Read the model definition and answer for the solid it produces. Units are mm, in the model's axes. Round coordinates to 2 decimals unless told otherwise and drop trailing zeros. Write each loop counter-clockwise with the first axis right and the second up, starting at its lowest first coordinate (ties: lowest second). Pieces come first, ordered by that corner, then holes. Notation, with made-up numbers: (45.25, 4) -> (63.25, 4) arc R9 ccw to (63.25, 12) -> close; hole circle Ø8 at (36, 24). An arc over 180 degrees is marked (long way). Return JSON: item names as keys, results as strings. Group by question number.
(1) A cutting plane is placed at D-D on y = 257. Give the vertices of the cut face in (x, z).
(2) A cutting plane is placed at A-A on x = -258.5. Give the vertices of the cut face in (y, z).
(3) Straight lines are drawn through the part: line 1 (X direction, y = 264, z = 1.8); line 2 (X direction, y = 268, z = 0.65); line 3 (X direction, y = 292, z = 2.3). For each, find the intervals that lie inside material, in ascending order.
(4) A cutting plane is placed at B-B on x = -199.5. Give the vertices of the cut face in (y, z), then the cut area to 3 significant figures.
(5) A cutting plane is placed at C-C on z = 1.3. State how many separate pieces and enclosed holes the cut face has, then the cut area to 3 significant figures.
(6) Given pin 1 (3 mm diameter, centred on x = -203.49, y = 292.5, fed in from +Z) (3 decimals); pin 2 (1.5 mm diameter, centred on x = -223.5, z = 1, fed in from +Y); pin 3 (1.5 mm diameter, centred on y = 314, z = 1, fed in from -X); pin 4 (1.5 mm diameter, centred on y = 309.5, z = 1.5, fed in from -X), each flat-ended and moving along its own axis, determine where each tip first touches the part or whether it passes through.
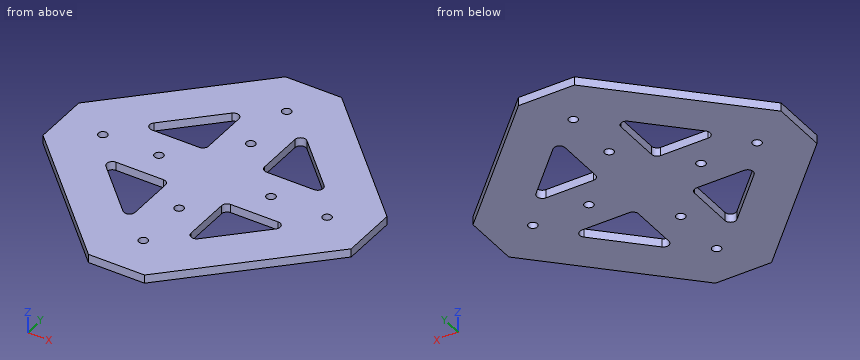
```python
from build123d import *

# Parameters (mm, degrees)
EXTRUDE1_DEPTH     = 3
SKETCH2_R          = 1.6
CUT_EXTRUDE1_DEPTH = 3
EXTRUDE2_DEPTH     = 10


with BuildPart() as part:
    # Sketch1 → Extrude1 (new body)
    with BuildSketch(Plane.XY):
        Polygon((-253.489921235, 347.497048214), (-233.489921235, 347.497048214), (-188.489921235, 302.497048214), (-188.489921235, 282.497048214), (-233.489921235, 237.497048214), (-253.489921235, 237.497048214), (-298.489921235, 282.497048214), (-298.489921235, 302.497048214), align=None)
    extrude(amount=EXTRUDE1_DEPTH)

    # Sketch2 → Cut-Extrude1 (cut)
    with BuildSketch(Plane.XY.offset(3)):
        with Locations((-203.489921235, 292.497048214)):
            Circle(SKETCH2_R)
        with Locations((-223.489921235, 292.497048214)):
            Circle(SKETCH2_R)
        with Locations((-243.489921235, 252.497048214)):
            Circle(SKETCH2_R)
        with Locations((-243.489921235, 272.497048214)):
            Circle(SKETCH2_R)
        with Locations((-283.489921235, 292.497048214)):
            Circle(SKETCH2_R)
        with Locations((-263.489921235, 292.497048214)):
            Circle(SKETCH2_R)
        with Locations((-243.489921235, 312.497048214)):
            Circle(SKETCH2_R)
        with Locations((-243.489921235, 332.497048214)):
            Circle(SKETCH2_R)
    extrude(amount=-CUT_EXTRUDE1_DEPTH, mode=Mode.SUBTRACT)

    # Sketch3 → Extrude2 (cut)
    with BuildSketch(Plane.XY.offset(3)):
        with BuildLine():
            Line((-256.904134797, 322.869631216), (-273.862504237, 305.911261776))
            ThreePointArc((-273.862504237, 305.911261776), (-274.29604974, 303.731681349), (-272.448290675, 302.497048214))
            Line((-272.448290675, 302.497048214), (-255.489921235, 302.497048214))
            ThreePointArc((-255.489921235, 302.497048214), (-254.075707673, 303.082834651), (-253.489921235, 304.497048214))
            Line((-253.489921235, 304.497048214), (-253.489921235, 321.455417653))
            ThreePointArc((-253.489921235, 321.455417653), (-254.72455437, 323.303176718), (-256.904134797, 322.869631216))
        make_face()
        with BuildLine():
            Line((-233.489921235, 304.497048214), (-233.489921235, 321.455417653))
            ThreePointArc((-233.489921235, 321.455417653), (-232.2552881, 323.303176718), (-230.075707673, 322.869631216))
            Line((-230.075707673, 322.869631216), (-213.117338233, 305.911261776))
            ThreePointArc((-213.117338233, 305.911261776), (-212.68379273, 303.731681349), (-214.531551795, 302.497048214))
            Line((-214.531551795, 302.497048214), (-231.489921235, 302.497048214))
            ThreePointArc((-231.489921235, 302.497048214), (-232.904134797, 303.082834651), (-233.489921235, 304.497048214))
        make_face()
        with BuildLine():
            Line((-230.075707673, 262.124465212), (-213.117338233, 279.082834651))
            ThreePointArc((-213.117338233, 279.082834651), (-212.68379273, 281.262415078), (-214.531551795, 282.497048214))
            Line((-214.531551795, 282.497048214), (-231.489921235, 282.497048214))
            ThreePointArc((-231.489921235, 282.497048214), (-232.904134797, 281.911261776), (-233.489921235, 280.497048214))
            Line((-233.489921235, 280.497048214), (-233.489921235, 263.538678774))
            ThreePointArc((-233.489921235, 263.538678774), (-232.2552881, 261.690919709), (-230.075707673, 262.124465212))
        make_face()
        with BuildLine():
            Line((-253.489921235, 280.497048214), (-253.489921235, 263.538678774))
            ThreePointArc((-253.489921235, 263.538678774), (-254.72455437, 261.690919709), (-256.904134797, 262.124465212))
            Line((-256.904134797, 262.124465212), (-273.862504237, 279.082834651))
            ThreePointArc((-273.862504237, 279.082834651), (-274.29604974, 281.262415078), (-272.448290675, 282.497048214))
            Line((-272.448290675, 282.497048214), (-255.489921235, 282.497048214))
            ThreePointArc((-255.489921235, 282.497048214), (-254.075707673, 281.911261776), (-253.489921235, 280.497048214))
        make_face()
    extrude(amount=-EXTRUDE2_DEPTH, mode=Mode.SUBTRACT)


solid = part.part
```
Checks:
{
 "1": {"outline": "(-272.99, 0) -> (-213.99, 0) -> (-213.99, 3) -> (-272.99, 3) -> close"},
 "2": {"outline": "(242.51, 0) -> (263.72, 0) -> (263.72, 3) -> (242.51, 3) -> close; (282.5, 0) -> (302.5, 0) -> (302.5, 3) -> (282.5, 3) -> close; (321.27, 0) -> (342.49, 0) -> (342.49, 3) -> (321.27, 3) -> close"},
 "3": {"line 1": "x = -279.99 to -258.78, -253.49 to -233.49, -228.2 to -206.99", "line 2": "x = -283.99 to -262.78, -253.49 to -233.49, -224.2 to -202.99", "line 3": "x = -298.49 to -285.01, -281.97 to -265.01, -261.97 to -225.01, -221.97 to -205.01, -201.97 to -188.49"},
 "4": {"outline": "(271.49, 0) -> (313.51, 0) -> (313.51, 3) -> (271.49, 3) -> close", "area": "126 mm^2"},
 "5": {"separate pieces": "1", "enclosed holes": "12", "area": "6,900 mm^2"},
 "6": {"pin 1": "passes through", "pin 2": "stops at y = 338.26", "pin 3": "stops at x = -287.74", "pin 4": "stops at x = -292.24"}
}
